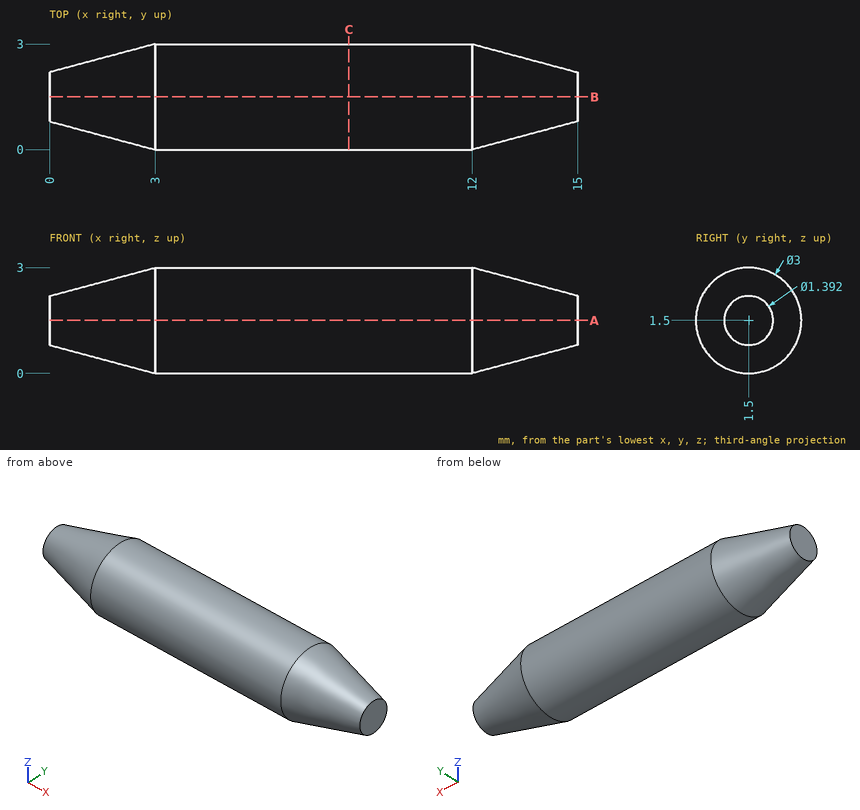
Input: dimensioned drawing with shaded views. Units: mm. Origin: part minimum x, y, z. Round coordinates to 2 decimals unless told otherwise and drop trailing zeros. Order: outer loops, then holes, each group sorted by start corner. A loop starts at its lowest first (then second) coordinate and runs counter-clockwise, first axis right, second up. Notation, with made-up numbers: (-19, -37) - (20, -37) arc R11 cw to (20, -30) - close; hole circle Ø3 at (43, -19.75). An arc over 180 degrees is marked (long way). Write item = value, one per line. Start each with the question number.
Q1. Cut plane C-C on x = 8.5. Return the cut outline in (y, z).
Q2. Cut plane A-A on z = 1.5. Return the cut outline in (x, y).
Q3. Ray query, line 1 (Y direction, x = 9.5, z = 1.05); line 2 (Z direction, x = 10.25, y = 1.9) (1 decimal); line 3 (Z direction, x = 3.5, y = 2.4). Return the intervals inside material, ascending. Write a range as from..to.
Outcome:
q1.outline = circle Ø3 at (1.5, 1.5)
q2.outline = (0, 0.8) - (3, 0) - (12, 0) - (15, 0.8) - (15, 2.2) - (12, 3) - (3, 3) - (0, 2.2) - close
q3.line_1 = 0.07..2.93
q3.line_2 = 0.1..2.9
q3.line_3 = 0.3..2.7
